Geometry: final body of the model. Coordinates: model frame, mm. Face numbers are marked on the shaded views. Coordinates: 2 decimals unless noted, no trailing zeros. Loops run counter-clockwise (first coordinate to the right, second up) from the corner with the lowest first, then second, coordinate; pieces in that order, holes last. Notation, with made-up numbers: (2.25, 2.25) -> (51.25, 2.25) arc R13 ccw to (51.25, 13.25) -> close; hole circle Ø9 at (12.25, 20). An arc over 180 degrees is marked (long way). One line per item, written item: value. Start each with the question number.
Item 1: Ray query, probe 1 along Z at (x, y) = (4.5, 1.5); probe 2 along Y at (x, z) = (2.5, 18.5); probe 3 along Z at (x, y) = (6.75, -22). Return the intervals inside material, ascending. Write a range as from..to.
Item 2: Section query C-C on x = -3.5. Return loops of the section in (y, z).
Item 3: Contact query for flat-ended pins moving along their axis: pin 1 Ø1 at (x, y) = (-2.5, 10) entering from -Z; pin 2 Ø23.5 at (y, z) = (0, 0) entering from +X; pin 3 Ø2 at (x, z) = (0.5, -19.5) entering from +Y; pin 4 Ø6 at (x, y) = (4, -16.5) entering from +Z. Output: stop coordinate, or through.
Item 4: Mould query, pull axis Z, two halves, no side actions, for the marked faces 1, 2 and 3. Classes: +Z half, -Z half, draft (parallel to the pull), parting line (faces both ways), or undercut.
Autodesk Inventor part; units mm, degrees
ref_plane "YZ Plane" through (0, 0, 0) normal (1, 0, 0) x (0, 1, 0)
ref_plane "XZ Plane" through (0, 0, 0) normal (0, 1, 0) x (-1, 0, 0)
ref_plane "XY Plane" through (0, 0, 0) normal (0, 0, 1) x (1, 0, 0)
sketch "Sketch1" plane through (0, 0, 0) normal (1, 0, 0) x (0, 1, 0)
  circle A0 centre (0, 0) radius 9
  circle A1 centre (0, 0) radius 27.5
  dimension "d1" = 18
  dimension "d2" = 55
extrude "Extrusion1" add sketch "Sketch1" along normal mid plane 16
sketch "Sketch2" plane through (8, 0, 0) normal (1, 0, 0) x (0, 0, -1)
  circle A0 centre (0, 0) radius 20
  circle A1 centre (0, 0) radius 24
  dimension "d5" = 48
  dimension "d6" = 40
extrude "Extrusion2" cut sketch "Sketch2" against normal blind 1
mirror "Mirror1" about plane through (0, 0, 0) normal (1, 0, 0) of "Extrusion2"
fillet "Fillet1" radius 1 4 edges at (8, -27.5, 0) (7, 0, 20) (-8, -27.5, 0) (-7, 0, 20)
properties part number "362-02"
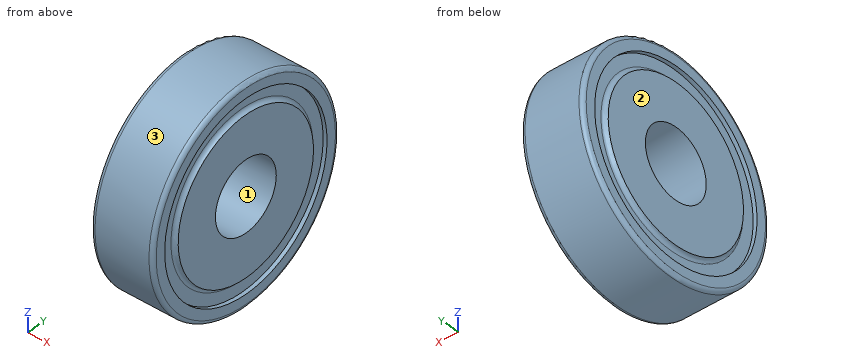
Reply:
1. probe 1: z = -27.46..-8.87, 8.87..27.46
1. probe 2: y = -20.35..20.35
1. probe 3: z = -16.5..16.5
2. outline: circle Ø55 at (0, 0); hole circle Ø18 at (0, 0)
3. pin 1: stops at z = -25.81
3. pin 2: stops at x = 8
3. pin 3: stops at y = 20.35
3. pin 4: stops at z = 23.96
4. face 1: undercut
4. face 2: draft
4. face 3: parting line
